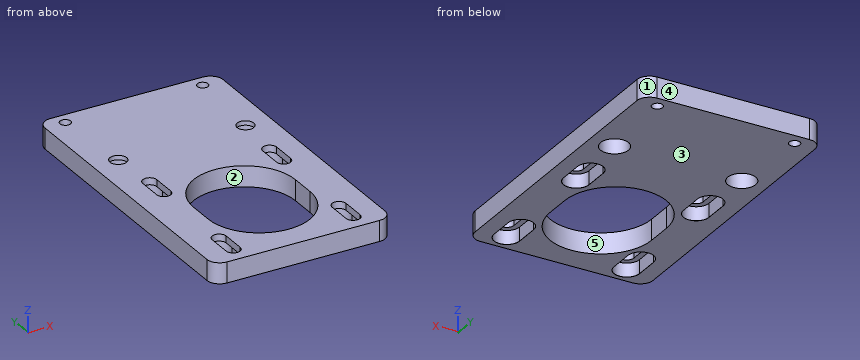
from build123d import *

# Parameters (mm, degrees)
BOSS_EXTRU_1_DEPTH                                 = 8
BOSS_EXTRU_1_DEPTH_BACK                            = 0.1
ESQUISSE1_W                                        = 70
ESQUISSE1_H                                        = 120
CHAMBRAGE_POUR_VIS_T_TE_HEXAGONALE_M62_D           = 6.6
CHAMBRAGE_POUR_VIS_T_TE_HEXAGONALE_M62_CBORE_D     = 11
CHAMBRAGE_POUR_VIS_T_TE_HEXAGONALE_M62_CBORE_DEPTH = 6.4
ESQUISSE4_R                                        = 20
ENL_V_MAT_EXTRU_1_DEPTH                            = 70.932896408
RAINURE_START                                      = -0.1
RAINURE_DE_CHAMBRAGE_POUR_VIS_T_TE_HEX_DEPTH       = 5.4
RAINURE_START_2                                    = 5.3
RAINURE_DE_CHAMBRAGE_POUR_VIS_T_TE_3_DEPTH         = 3.7
TROU_POUR_TARAUDAGE_POUR_TROU_TARAUD_M5_D          = 4.2
CONG_1_R                                           = 5


with BuildPart() as part:
    # Esquisse1 → Boss.-Extru.1 (new, two sides: drawn at the far end of the back side and taken through both)
    with BuildSketch(Plane.XY.offset(-BOSS_EXTRU_1_DEPTH_BACK)):
        Rectangle(ESQUISSE1_W, ESQUISSE1_H)
    extrude(amount=BOSS_EXTRU_1_DEPTH + BOSS_EXTRU_1_DEPTH_BACK)

    # Chambrage pour vis à tête hexagonale M62 (through all)
    with Locations(Plane(origin=(0, 0, -0.1), x_dir=(-1, 0, 0), z_dir=(0, 0, -1))):
        with Locations((25, 22.5), (-25, 22.5)):
            CounterBoreHole(CHAMBRAGE_POUR_VIS_T_TE_HEXAGONALE_M62_D / 2, CHAMBRAGE_POUR_VIS_T_TE_HEXAGONALE_M62_CBORE_D / 2, CHAMBRAGE_POUR_VIS_T_TE_HEXAGONALE_M62_CBORE_DEPTH)

    # Esquisse4 → Enlèv. mat.-Extru.1 (cut, through all)
    with BuildSketch(Plane.XY.offset(8)):
        with Locations((0, -20)):
            Circle(ESQUISSE4_R)
        with BuildLine():
            Line((20, -30), (20, -20))
            ThreePointArc((20, -20), (0, -40), (-20, -20))
            Line((-20, -20), (-20, -30))
            ThreePointArc((-20, -30), (0, -50), (20, -30))
        make_face()
    extrude(amount=-ENL_V_MAT_EXTRU_1_DEPTH, mode=Mode.SUBTRACT)

    # Rainure de chambrage pour vis à tête hexagonale M53: read off the stored shape, not the designer's step
    # Rainure de chambrage pour vis _ t_te 2 → Rainure de chambrage pour vis à tête hexagonale M53 (cut)
    with BuildSketch(Plane.XY.offset(RAINURE_START)):
        with BuildLine():
            ThreePointArc((-18.57, 3.57), (-23.57, 8.57), (-28.57, 3.57))
            Line((-28.57, 3.57), (-28.57, -5.93))
            ThreePointArc((-28.57, -5.93), (-23.57, -10.93), (-18.57, -5.93))
            Line((-18.57, -5.93), (-18.57, 3.57))
        make_face()
        with BuildLine():
            Line((-18.57, -53.07), (-18.57, -43.57))
            ThreePointArc((-18.57, -43.57), (-23.57, -38.57), (-28.57, -43.57))
            Line((-28.57, -43.57), (-28.57, -53.07))
            ThreePointArc((-28.57, -53.07), (-23.57, -58.07), (-18.57, -53.07))
        make_face()
        with BuildLine():
            ThreePointArc((28.57, -43.57), (23.57, -38.57), (18.57, -43.57))
            Line((18.57, -43.57), (18.57, -53.07))
            ThreePointArc((18.57, -53.07), (23.57, -58.07), (28.57, -53.07))
            Line((28.57, -53.07), (28.57, -43.57))
        make_face()
        with BuildLine():
            Line((28.57, -5.93), (28.57, 3.57))
            ThreePointArc((28.57, 3.57), (23.57, 8.57), (18.57, 3.57))
            Line((18.57, 3.57), (18.57, -5.93))
            ThreePointArc((18.57, -5.93), (23.57, -10.93), (28.57, -5.93))
        make_face()
    extrude(amount=RAINURE_DE_CHAMBRAGE_POUR_VIS_T_TE_HEX_DEPTH, mode=Mode.SUBTRACT)

    # Rainure de chambrage pour vis _ t_te 3 o → Rainure de chambrage pour vis _ t_te 3 (cut)
    with BuildSketch(Plane.XY.offset(RAINURE_START_2)):
        with BuildLine():
            ThreePointArc((-20.82, 3.57), (-23.57, 6.32), (-26.32, 3.57))
            Line((-26.32, 3.57), (-26.32, -5.93))
            ThreePointArc((-26.32, -5.93), (-23.57, -8.68), (-20.82, -5.93))
            Line((-20.82, -5.93), (-20.82, 3.57))
        make_face()
        with BuildLine():
            Line((-20.82, -53.07), (-20.82, -43.57))
            ThreePointArc((-20.82, -43.57), (-23.57, -40.82), (-26.32, -43.57))
            Line((-26.32, -43.57), (-26.32, -53.07))
            ThreePointArc((-26.32, -53.07), (-23.57, -55.82), (-20.82, -53.07))
        make_face()
        with BuildLine():
            ThreePointArc((26.32, -43.57), (23.57, -40.82), (20.82, -43.57))
            Line((20.82, -43.57), (20.82, -53.07))
            ThreePointArc((20.82, -53.07), (23.57, -55.82), (26.32, -53.07))
            Line((26.32, -53.07), (26.32, -43.57))
        make_face()
        with BuildLine():
            Line((26.32, -5.93), (26.32, 3.57))
            ThreePointArc((26.32, 3.57), (23.57, 6.32), (20.82, 3.57))
            Line((20.82, 3.57), (20.82, -5.93))
            ThreePointArc((20.82, -5.93), (23.57, -8.68), (26.32, -5.93))
        make_face()
    extrude(amount=RAINURE_DE_CHAMBRAGE_POUR_VIS_T_TE_3_DEPTH, mode=Mode.SUBTRACT)

    # Rainure de chambrage pour vis _ t_te 4: loft between two sections, ruled curve by curve
    rainure_de_chambrage_pour_vis_t_te_4_from = [
        Edge.make_three_point_arc((-28.57, 3.57, -0.075), (-27.105533906, 7.105533906, -0.075), (-23.57, 8.57, -0.075)),
        Edge.make_three_point_arc((-23.57, 8.57, -0.075), (-20.034466094, 7.105533906, -0.075), (-18.57, 3.57, -0.075)),
        Edge.make_three_point_arc((-18.57, -5.93, -0.075), (-20.034466094, -9.465533906, -0.075), (-23.57, -10.93, -0.075)),
        Edge.make_three_point_arc((-23.57, -10.93, -0.075), (-27.105533906, -9.465533906, -0.075), (-28.57, -5.93, -0.075)),
        Edge.make_line((-18.57, 3.57, -0.075), (-18.57, -5.93, -0.075)),
        Edge.make_line((-28.57, 3.57, -0.075), (-28.57, -5.93, -0.075)),
    ]
    rainure_de_chambrage_pour_vis_t_te_4_to = [
        Edge.make_three_point_arc((-28.595, 3.57, -0.1), (-27.123211575, 7.123211575, -0.1), (-23.57, 8.595, -0.1)),
        Edge.make_three_point_arc((-23.57, 8.595, -0.1), (-20.016788425, 7.123211575, -0.1), (-18.545, 3.57, -0.1)),
        Edge.make_three_point_arc((-18.545, -5.93, -0.1), (-20.016788425, -9.483211575, -0.1), (-23.57, -10.955, -0.1)),
        Edge.make_three_point_arc((-23.57, -10.955, -0.1), (-27.123211575, -9.483211575, -0.1), (-28.595, -5.93, -0.1)),
        Edge.make_line((-18.545, 3.57, -0.1), (-18.545, -5.93, -0.1)),
        Edge.make_line((-28.595, 3.57, -0.1), (-28.595, -5.93, -0.1)),
    ]
    rainure_de_chambrage_pour_vis_t_te_4 = Solid(Shell([*[Face.make_surface_from_curves(rainure_de_chambrage_pour_vis_t_te_4_from[k], rainure_de_chambrage_pour_vis_t_te_4_to[k]) for k in range(6)], Face(Wire(rainure_de_chambrage_pour_vis_t_te_4_from)), Face(Wire(rainure_de_chambrage_pour_vis_t_te_4_to))]))
    add(rainure_de_chambrage_pour_vis_t_te_4, mode=Mode.SUBTRACT)

    # Rainure de chambrage pour vis _ t_te 5: loft between two sections, ruled curve by curve
    rainure_de_chambrage_pour_vis_t_te_5_from = [
        Edge.make_three_point_arc((-28.57, -43.57, -0.075), (-27.105533906, -40.034466094, -0.075), (-23.57, -38.57, -0.075)),
        Edge.make_three_point_arc((-23.57, -38.57, -0.075), (-20.034466094, -40.034466094, -0.075), (-18.57, -43.57, -0.075)),
        Edge.make_three_point_arc((-18.57, -53.07, -0.075), (-20.034466094, -56.605533906, -0.075), (-23.57, -58.07, -0.075)),
        Edge.make_three_point_arc((-23.57, -58.07, -0.075), (-27.105533906, -56.605533906, -0.075), (-28.57, -53.07, -0.075)),
        Edge.make_line((-18.57, -43.57, -0.075), (-18.57, -53.07, -0.075)),
        Edge.make_line((-28.57, -43.57, -0.075), (-28.57, -53.07, -0.075)),
    ]
    rainure_de_chambrage_pour_vis_t_te_5_to = [
        Edge.make_three_point_arc((-28.595, -43.57, -0.1), (-27.123211575, -40.016788425, -0.1), (-23.57, -38.545, -0.1)),
        Edge.make_three_point_arc((-23.57, -38.545, -0.1), (-20.016788425, -40.016788425, -0.1), (-18.545, -43.57, -0.1)),
        Edge.make_three_point_arc((-18.545, -53.07, -0.1), (-20.016788425, -56.623211575, -0.1), (-23.57, -58.095, -0.1)),
        Edge.make_three_point_arc((-23.57, -58.095, -0.1), (-27.123211575, -56.623211575, -0.1), (-28.595, -53.07, -0.1)),
        Edge.make_line((-18.545, -43.57, -0.1), (-18.545, -53.07, -0.1)),
        Edge.make_line((-28.595, -43.57, -0.1), (-28.595, -53.07, -0.1)),
    ]
    rainure_de_chambrage_pour_vis_t_te_5 = Solid(Shell([*[Face.make_surface_from_curves(rainure_de_chambrage_pour_vis_t_te_5_from[k], rainure_de_chambrage_pour_vis_t_te_5_to[k]) for k in range(6)], Face(Wire(rainure_de_chambrage_pour_vis_t_te_5_from)), Face(Wire(rainure_de_chambrage_pour_vis_t_te_5_to))]))
    add(rainure_de_chambrage_pour_vis_t_te_5, mode=Mode.SUBTRACT)

    # Rainure de chambrage pour vis _ t_te 6: loft between two sections, ruled curve by curve
    rainure_de_chambrage_pour_vis_t_te_6_from = [
        Edge.make_three_point_arc((18.57, -43.57, -0.075), (20.034466094, -40.034466094, -0.075), (23.57, -38.57, -0.075)),
        Edge.make_three_point_arc((23.57, -38.57, -0.075), (27.105533906, -40.034466094, -0.075), (28.57, -43.57, -0.075)),
        Edge.make_three_point_arc((28.57, -53.07, -0.075), (27.105533906, -56.605533906, -0.075), (23.57, -58.07, -0.075)),
        Edge.make_three_point_arc((23.57, -58.07, -0.075), (20.034466094, -56.605533906, -0.075), (18.57, -53.07, -0.075)),
        Edge.make_line((28.57, -43.57, -0.075), (28.57, -53.07, -0.075)),
        Edge.make_line((18.57, -43.57, -0.075), (18.57, -53.07, -0.075)),
    ]
    rainure_de_chambrage_pour_vis_t_te_6_to = [
        Edge.make_three_point_arc((18.545, -43.57, -0.1), (20.016788425, -40.016788425, -0.1), (23.57, -38.545, -0.1)),
        Edge.make_three_point_arc((23.57, -38.545, -0.1), (27.123211575, -40.016788425, -0.1), (28.595, -43.57, -0.1)),
        Edge.make_three_point_arc((28.595, -53.07, -0.1), (27.123211575, -56.623211575, -0.1), (23.57, -58.095, -0.1)),
        Edge.make_three_point_arc((23.57, -58.095, -0.1), (20.016788425, -56.623211575, -0.1), (18.545, -53.07, -0.1)),
        Edge.make_line((28.595, -43.57, -0.1), (28.595, -53.07, -0.1)),
        Edge.make_line((18.545, -43.57, -0.1), (18.545, -53.07, -0.1)),
    ]
    rainure_de_chambrage_pour_vis_t_te_6 = Solid(Shell([*[Face.make_surface_from_curves(rainure_de_chambrage_pour_vis_t_te_6_from[k], rainure_de_chambrage_pour_vis_t_te_6_to[k]) for k in range(6)], Face(Wire(rainure_de_chambrage_pour_vis_t_te_6_from)), Face(Wire(rainure_de_chambrage_pour_vis_t_te_6_to))]))
    add(rainure_de_chambrage_pour_vis_t_te_6, mode=Mode.SUBTRACT)

    # Rainure de chambrage pour vis _ t_te 7: loft between two sections, ruled curve by curve
    rainure_de_chambrage_pour_vis_t_te_7_from = [
        Edge.make_three_point_arc((18.57, 3.57, -0.075), (20.034466094, 7.105533906, -0.075), (23.57, 8.57, -0.075)),
        Edge.make_three_point_arc((23.57, 8.57, -0.075), (27.105533906, 7.105533906, -0.075), (28.57, 3.57, -0.075)),
        Edge.make_three_point_arc((28.57, -5.93, -0.075), (27.105533906, -9.465533906, -0.075), (23.57, -10.93, -0.075)),
        Edge.make_three_point_arc((23.57, -10.93, -0.075), (20.034466094, -9.465533906, -0.075), (18.57, -5.93, -0.075)),
        Edge.make_line((28.57, 3.57, -0.075), (28.57, -5.93, -0.075)),
        Edge.make_line((18.57, 3.57, -0.075), (18.57, -5.93, -0.075)),
    ]
    rainure_de_chambrage_pour_vis_t_te_7_to = [
        Edge.make_three_point_arc((18.545, 3.57, -0.1), (20.016788425, 7.123211575, -0.1), (23.57, 8.595, -0.1)),
        Edge.make_three_point_arc((23.57, 8.595, -0.1), (27.123211575, 7.123211575, -0.1), (28.595, 3.57, -0.1)),
        Edge.make_three_point_arc((28.595, -5.93, -0.1), (27.123211575, -9.483211575, -0.1), (23.57, -10.955, -0.1)),
        Edge.make_three_point_arc((23.57, -10.955, -0.1), (20.016788425, -9.483211575, -0.1), (18.545, -5.93, -0.1)),
        Edge.make_line((28.595, 3.57, -0.1), (28.595, -5.93, -0.1)),
        Edge.make_line((18.545, 3.57, -0.1), (18.545, -5.93, -0.1)),
    ]
    rainure_de_chambrage_pour_vis_t_te_7 = Solid(Shell([*[Face.make_surface_from_curves(rainure_de_chambrage_pour_vis_t_te_7_from[k], rainure_de_chambrage_pour_vis_t_te_7_to[k]) for k in range(6)], Face(Wire(rainure_de_chambrage_pour_vis_t_te_7_from)), Face(Wire(rainure_de_chambrage_pour_vis_t_te_7_to))]))
    add(rainure_de_chambrage_pour_vis_t_te_7, mode=Mode.SUBTRACT)

    # Trou pour taraudage pour trou taraudé M51 (through all)
    with Locations(Plane(origin=(0, 0, -0.1), x_dir=(-1, 0, 0), z_dir=(0, 0, -1))):
        with Locations((-27, 55), (27, 55)):
            Hole(TROU_POUR_TARAUDAGE_POUR_TROU_TARAUD_M5_D / 2)

    # Congé1
    cong_1_edges = [part.edges().sort_by_distance(p)[0] for p in [
        (35, -60, 3.95),
        (-35, -60, 3.95),
        (-35, 60, 3.95),
        (35, 60, 3.95),
    ]]
    fillet(cong_1_edges, radius=CONG_1_R)


solid = part.part
Verification items for the finished model (mm, model axes). Face numbers are marked on the shaded views. A direction names the side the tool comes from. Coordinates: 2 decimals unless noted, no trailing zeros. Order: outer loops, then holes, each group sorted by start corner. A loop starts at its lowest first (then second) coordinate and runs counter-clockwise, first axis right, second up. Notation, with made-up numbers: M 8,-18 L 53,-18 A24 ccw 53,-8 Z; hole C 37.5,47 d9. An arc over 180 degrees is marked long. Write each question's results on one line, items separated by ' | '.
1) Section check A-A on z = 4. Give the number of separate pieces and of enclosed holes in the cut face, plus the area to 3 significant figures.
Solved:
separate pieces: 1 | enclosed holes: 9 | area: 5,810 mm²
2) Release check for a two-part mould opening along Y. For the marked faces 1, 2 and 3 record: pulls with the +Y half, pulls with the -Y half, needs draft (parallel to the pull), parting line crosses it, or undercut.
Solved:
face 1: pulls with the +Y half | face 2: undercut | face 3: needs draft
3) Scan lines: line 1 along X through (y, z) = (4, 2.5); line 2 along X through (y, z) = (1, 7.5); line 3 along Y through (x, z) = (23, 7). Record each from-to range of solid material in increasing order. Write a range as [from, to].
Solved:
line 1: x = [-35, -28.55], [-18.59, 18.59], [28.55, 35] | line 2: x = [-35, -26.32], [-20.82, 20.82], [26.32, 35] | line 3: y = [-60, -55.76], [-40.88, -8.62], [6.26, 19.88], [25.12, 60]
4) Section check C-C on x = -4.5. Record the cut outline in (y, z), plus the area to 3 significant figures.
Solved:
outline: M -60,-0.1 L -49.49,-0.1 L -49.49,8 L -60,8 Z; M -0.51,-0.1 L 60,-0.1 L 60,8 L -0.51,8 Z | area: 575 mm²
5) Gauge pin test, flat ends, axial feed: pin 1 Ø6 at (x, y) = (25, 22.5) entering from +Z; pin 2 Ø5 at (x, y) = (25.5, -1.5) entering from -Z. Record the tip position at first contact, or that the pin passes through.
Solved:
pin 1: passes through | pin 2: stops at z = 5.3
6) Access from +Z, -Z, +X, -X, +Y, -Y to the whole of each face (thin tool, end or side, straight path). Record for the marked faces 4 and 5.
Solved:
face 4: +Z, -Z, +X, -X, +Y | face 5: +Z, -Z
7) Section check D-D on y = -35.5. Record the cut outline in (x, z).
Solved:
outline: M -35,-0.1 L -19.23,-0.1 L -19.23,8 L -35,8 Z; M 19.23,-0.1 L 35,-0.1 L 35,8 L 19.23,8 Z
8) Section check B-B on y = 22.5. Record the cut outline in (x, z), plus the area to 3 significant figures.
Solved:
outline: M -35,-0.1 L -30.5,-0.1 L -30.5,6.3 L -28.3,6.3 L -28.3,8 L -35,8 Z; M -21.7,6.3 L -19.5,6.3 L -19.5,-0.1 L 19.5,-0.1 L 19.5,6.3 L 21.7,6.3 L 21.7,8 L -21.7,8 Z; M 28.3,6.3 L 30.5,6.3 L 30.5,-0.1 L 35,-0.1 L 35,8 L 28.3,8 Z | area: 404 mm²
